from build123d import *

# Parameters (mm, degrees)
SKETCH1_W           = 177.8
SKETCH1_H           = 127
SKETCH1_R           = 5.588
SKETCH1_R_2         = 1.4605
SKETCH1_W_2         = 28.956
SKETCH1_H_2         = 59.69
BOSS_EXTRUDE1_DEPTH = 12.7
SKETCH3_W           = 8.128
SKETCH3_H           = 35.052
SKETCH3_W_2         = 5.08
SKETCH3_H_2         = 10.16
CUT_EXTRUDE3_DEPTH  = 13.7


with BuildPart() as part:
    # Sketch1 → Boss-Extrude1 (new body)
    with BuildSketch(Plane(origin=(0, 0, 0), x_dir=(1, 0, 0), z_dir=(0, 1, 0))):
        Rectangle(SKETCH1_W, SKETCH1_H)
        with Locations((-19.05, 0)):
            Circle(SKETCH1_R, mode=Mode.SUBTRACT)
        with Locations((49.825565695, -32.301655548)):
            Circle(SKETCH1_R_2, mode=Mode.SUBTRACT)
        with Locations((65.700565695, -32.301655548)):
            Circle(SKETCH1_R_2, mode=Mode.SUBTRACT)
        with Locations((49.825565695, 35.719544452)):
            Circle(SKETCH1_R_2, mode=Mode.SUBTRACT)
        with Locations((65.700565695, 35.719544452)):
            Circle(SKETCH1_R_2, mode=Mode.SUBTRACT)
        with Locations((57.763065695, 1.908969452)):
            Rectangle(SKETCH1_W_2, SKETCH1_H_2, mode=Mode.SUBTRACT)
    extrude(amount=BOSS_EXTRUDE1_DEPTH)

    # Sketch3 → Cut-Extrude3 (cut, through all)
    with BuildSketch(Plane(origin=(0, 0, 0), x_dir=(1, 0, 0), z_dir=(0, 1, 0))):
        with Locations((39.301988782, -14.045405548)):
            Rectangle(SKETCH3_W, SKETCH3_H)
        with Locations((76.224142608, -14.045405548)):
            Rectangle(SKETCH3_W, SKETCH3_H)
        with Locations((57.763065695, -33.016030548)):
            Rectangle(SKETCH3_W_2, SKETCH3_H_2)
        with Locations((57.763065695, 36.833969452)):
            Rectangle(SKETCH3_W_2, SKETCH3_H_2)
    extrude(amount=CUT_EXTRUDE3_DEPTH, mode=Mode.SUBTRACT)


solid = part.part
Could you check a few things on this model? Use its own coordinates, in mm. A direction names the side the tool comes from. Coordinates: 2 decimals unless noted, no trailing zeros. Order: outer loops, then holes, each group sorted by start corner. A loop starts at its lowest first (then second) coordinate and runs counter-clockwise, first axis right, second up. Notation, with made-up numbers: (0.25, 30.25) - (19.25, 30.25) arc R32 cw to (19.25, 67.25) - close; hole circle Ø4 at (-15.75, 71.25). An arc over 180 degrees is marked (long way). Answer in a Markdown table with one row per item. Add a question column.
(1) Will this pin go through, and if not, where does the flat tip stop? pin 1 (4.5 mm diameter, centred on x = 65.7, z = -35.72, fed in from +Y).
(2) If we section it at A-A, the plane z = 0: Please give me the cut outline in (x, y).
(3) I need wall thicknesses on L1, parallel to X at y = 1, z = 28; L2, parallel to Z at x = -19.05, y = 5; L3, parallel to X at y = 6, z = -34. Which ranges of each line are inside material? Lowest first, please.
(4) If we section it at D-D, the plane y = 5.5: State how many separate pieces and enclosed holes the cut face has, then the cut area to 3 significant figures.
(5) On a 3-axis mill with a long thin cutter (end or side, diameter ignored), from which of +Z, -Z, +X, -X, +Y, -Y can I reach the whole of each face in a straight line? I mean faces 5 (the face through (39, 6, 31.571)), 6 (the face through (-1, 12.7, -1)). Say none if no direction works.
(6) If we mould it in two halves opening along Z, with no side actions, what happens to faces 1 (the face through (-1, 6, 63.5)), 2 (the face through (-1, 0, -1)), 3 (the face through (72.16, 6, 30)), 4 (the face through (-1, 6, -63.5))? For each: released by +Z, released by -Z, zero draft, split by the parting line, or undercut.
(7) If we section it at C-C, the plane z = -19: Please give me the cut outline in (x, y).
(8) If we section it at B-B, the plane x = -19.05: Please give me the cut outline in (y, z), then the cut area to 3 significant figures.
Results are:
| question | item | result |
|---|---|---|
| 1 | pin 1 | stops at y = 12.7 |
| 2 | outline | (-88.9, 0) - (-24.64, 0) - (-24.64, 12.7) - (-88.9, 12.7) - close; (-13.46, 0) - (35.24, 0) - (35.24, 12.7) - (-13.46, 12.7) - close; (80.29, 0) - (88.9, 0) - (88.9, 12.7) - (80.29, 12.7) - close |
| 3 | L1 | x = -88.9 to 35.24, 43.37 to 55.22, 60.3 to 72.16, 80.29 to 88.9 |
| 3 | L2 | z = -63.5 to -5.59, 5.59 to 63.5 |
| 3 | L3 | x = -88.9 to 55.22, 60.3 to 88.9 |
| 4 | separate pieces | 1 |
| 4 | enclosed holes | 6 |
| 4 | area | 20,100 mm2 |
| 5 | face 5 | +Y, -Y |
| 5 | face 6 | +Z, -Z, +X, -X, +Y |
| 6 | face 1 | released by +Z |
| 6 | face 2 | zero draft |
| 6 | face 3 | undercut |
| 6 | face 4 | released by -Z |
| 7 | outline | (-88.9, 0) - (43.29, 0) - (43.29, 12.7) - (-88.9, 12.7) - close; (72.24, 0) - (88.9, 0) - (88.9, 12.7) - (72.24, 12.7) - close |
| 8 | outline | (0, -63.5) - (12.7, -63.5) - (12.7, -5.59) - (0, -5.59) - close; (0, 5.59) - (12.7, 5.59) - (12.7, 63.5) - (0, 63.5) - close |
| 8 | area | 1,470 mm2 |
